```python
from build123d import *

# Parameters (mm, degrees)
F1_DEPTH = 255.5875
F3_DEPTH = 12.7
F5_DEPTH = 12.7


with BuildPart() as f1:
    # F0 (on Top) → F1 (new body)
    with BuildSketch(Plane.XY):
        with BuildLine():
            ThreePointArc((12.7, 6.35), (10.840128, 10.840128), (6.35, 12.7))
            Line((6.35, 12.7), (-6.35, 12.7))
            ThreePointArc((-6.35, 12.7), (-10.840128, 10.840128), (-12.7, 6.35))
            Line((-12.7, 6.35), (-12.7, -6.35))
            ThreePointArc((-12.7, -6.35), (-10.840128, -10.840128), (-6.35, -12.7))
            Line((-6.35, -12.7), (6.35, -12.7))
            ThreePointArc((6.35, -12.7), (10.840128, -10.840128), (12.7, -6.35))
            Line((12.7, -6.35), (12.7, 6.35))
        make_face()
    extrude(amount=F1_DEPTH)

    # F2 (on Right) → F3 (cut, symmetric)
    with BuildSketch(Plane.YZ):
        Polygon((-17.71266, 0), (12.69978, 0), (-17.71266, 2.660744), align=None)
    extrude(amount=F3_DEPTH, both=True, mode=Mode.SUBTRACT)

    # F4 (on Right) → F5 (cut, symmetric)
    with BuildSketch(Plane.YZ):
        Polygon((-13.445419, 253.380933), (13.181062, 255.710448), (-13.445419, 255.710448), align=None)
    extrude(amount=F5_DEPTH, both=True, mode=Mode.SUBTRACT)


solid = f1.part
```
Verification items for the finished model (mm, model axes). Round coordinates to 2 decimals unless told otherwise and drop trailing zeros. Order: outer loops, then holes, each group sorted by start corner. A loop starts at its lowest first (then second) coordinate and runs counter-clockwise, first axis right, second up. Notation, with made-up numbers: (8.5, 50) - (47.5, 50) arc R24 cw to (47.5, 69) - close; hole circle Ø8 at (69.25, 14.25). An arc over 180 degrees is marked (long way). Use CSV: the item, a comma, the result in double quotes. Start each with the question number.
1) Section check A-A, the plane z = 80.5. Record the cut outline in (x, y), plus the area to 3 significant figures.
2) Section check C-C, the plane y = -10. Record the cut outline in (x, z).
3) Thickness scan on L1, parallel to Y at x = -6.5, z = 104.5; L2, parallel to Z at x = 3, y = -8.5; L3, parallel to Z at x = 2.5, y = 0. Record the ranges inside material, lowest first.
4) Section check B-B, the plane y = 9. Record the cut outline in (x, z), plus the area to 3 significant figures.
5) Go/stop test with flat-tipped pins: P1, Ø6, axis at x = -9.5, z = 224.5, coming from the -Y side; P2, Ø2, axis at y = 10, z = 32.5, coming from the -X side; P3, Ø6, axis at x = 2.5, y = -3.5, coming from the +Z side. Record where each tip stops, or that it passes through.
Answers:
1,outline,"(-12.7, -6.35) arc R6.35 ccw to (-6.35, -12.7) - (6.35, -12.7) arc R6.35 ccw to (12.7, -6.35) - (12.7, 6.35) arc R6.35 ccw to (6.35, 12.7) - (-6.35, 12.7) arc R6.35 ccw to (-12.7, 6.35) - close"
1,area,"611 mm²"
2,outline,"(-11.55, 1.99) - (11.55, 1.99) - (11.55, 253.68) - (-11.55, 253.68) - close"
3,L1,"y = -12.7 to 12.7"
3,L2,"z = 1.85 to 253.81"
3,L3,"z = 1.11 to 254.56"
4,outline,"(-12.12, 0.32) - (12.12, 0.32) - (12.12, 255.34) - (-12.12, 255.34) - close"
4,area,"6,180 mm²"
5,P1,"stops at y = -12.7"
5,P2,"stops at x = -12.12"
5,P3,"stops at z = 254.51"
